```python
from build123d import *

# Parameters (mm, degrees)
F0_W     = 67.1
F0_H     = 138.3
F1_DEPTH = 3.55
F2_T     = -2.54
F3_R     = 5.08
F4_W     = 18.64754
F4_H     = 6.885249
F5_DEPTH = 12.5


with BuildPart() as f1:
    # F0 (on Front) → F1 (new body, symmetric)
    with BuildSketch(Plane.XZ):
        Rectangle(F0_W, F0_H)
    extrude(amount=F1_DEPTH, both=True)

    # F2
    f2_openings = [f1.faces().sort_by_distance(p)[0] for p in [
        (0, -3.55, 0),
    ]]
    offset(amount=F2_T, openings=f2_openings)

    # F3
    f3_edges = [f1.edges().sort_by_distance(p)[0] for p in [
        (33.55, 0, 69.15),
        (-33.55, 0, 69.15),
        (-33.55, 0, -69.15),
        (33.55, 0, -69.15),
    ]]
    fillet(f3_edges, radius=F3_R)

    # F4 (on Front) → F5 (cut, symmetric)
    with BuildSketch(Plane.XZ):
        with Locations((19.651639, 59.241807)):
            Rectangle(F4_W, F4_H)
    extrude(amount=F5_DEPTH, both=True, mode=Mode.SUBTRACT)


solid = f1.part
```
The model under review builds one solid part; all positions refer to its coordinate system, in mm. A direction names the side the tool comes from. Round coordinates to 2 decimals unless told otherwise and drop trailing zeros. Write each loop counter-clockwise with the first axis right and the second up, starting at its lowest first coordinate (ties: lowest second). Pieces come first, ordered by that corner, then holes. Notation, with made-up numbers: M -28,46.5 L 23,46.5 A18 cw 23,81.5 Z; hole C -18.75,45 d6. An arc over 180 degrees is marked long. Use CSV: the item, a comma, the result in double quotes. Start each with the question number.
(1) For line 1 along Z through (x, y) = (14.5, -2.5); line 2 along X through (y, z) = (-1.75, -9); line 3 along Y through (x, z) = (-22, 41), list the stretches that pass through material, from the lowest coordinate up.
(2) We need section B-B, the plane z = 61. State the section outline as (x, y) points.
(3) We need section D-D, the plane z = 6. State the section outline as (x, y) points.
(4) Tool access review of faces 1 (the face through (20, 2, 55.799)), 2 (the face through (0, 3.55, 1)), 3 (the face through (31.01, -1, -1)): name each direction out of +Z, -Z, +X, -X, +Y, -Y from which nothing blocks a thin tool from reaching the whole face with its end or side.
(5) Clearance check with a flat-ended pin moving along its axis: P1, Ø18.5, axis at x = 6, z = 19.5, coming from the -Y side. State where the tip first meets the part, or that it passes through.
(6) We need section A-A, the plane y = -1.75. State the section outline as (x, z) points.
(7) The part is to be moulded in two halves that separate along X. For faces 4 (the face through (0, 1.01, 1)), 5 (the face through (10.328, 2, 59)), 6 (the face through (0, 0, -69.15)), 7 (the face through (32.101, 0.05, 67.622)), say which applies: +X half, -X half, draft (parallel to the pull), parting line (faces both ways), or undercut.
(8) We need section C-C, the plane x = -20. State the section outline as (y, z) points, then the cut area to 3 significant figures.
Findings:
1,line 1,"-69.15 to -66.61, 66.61 to 69.15"
1,line 2,"-33.55 to -31.01, 31.01 to 33.55"
1,line 3,"1.01 to 3.55"
2,outline,"M -33.55,-3.55 L -31.01,-3.55 L -31.01,1.01 L 10.33,1.01 L 10.33,3.55 L -33.55,3.55 Z; M 28.98,1.01 L 31.01,1.01 L 31.01,-3.55 L 33.55,-3.55 L 33.55,3.55 L 28.98,3.55 Z"
3,outline,"M -33.55,-3.55 L -31.01,-3.55 L -31.01,1.01 L 31.01,1.01 L 31.01,-3.55 L 33.55,-3.55 L 33.55,3.55 L -33.55,3.55 Z"
4,face 1,"+Y, -Y"
4,face 2,"+Z, -Z, +X, -X, +Y"
4,face 3,"-Y"
5,P1,"y = 1.01"
6,outline,"M -33.55,-64.07 A5.08 ccw -28.47,-69.15 L 28.47,-69.15 A5.08 ccw 33.55,-64.07 L 33.55,64.07 A5.08 ccw 28.47,69.15 L -28.47,69.15 A5.08 ccw -33.55,64.07 Z; hole M -31.01,-66.61 L 31.01,-66.61 L 31.01,66.61 L -31.01,66.61 Z"
7,face 4,"undercut"
7,face 5,"undercut"
7,face 6,"draft"
7,face 7,"+X half"
8,outline,"M -3.55,-69.15 L 3.55,-69.15 L 3.55,69.15 L -3.55,69.15 L -3.55,66.61 L 1.01,66.61 L 1.01,-66.61 L -3.55,-66.61 Z"
8,area,"374 mm^2"
